Autodesk Inventor part; units mm, degrees
ref_plane "YZ Plane" through (0, 0, 0) normal (1, 0, 0) x (0, 1, 0)
ref_plane "XZ Plane" through (0, 0, 0) normal (0, 1, 0) x (-1, 0, 0)
ref_plane "XY Plane" through (0, 0, 0) normal (0, 0, 1) x (1, 0, 0)
sketch "Эскиз1" plane through (0, 0, 0) normal (0, 0, 1) x (1, 0, 0)
  arc A0 (0.9499, 0.3125) -> (0.1, 0.995) centre (0, 0) ccw
  line L0 (0.9499, 0.3125) -> (1.4499, 0.3125)
  line L1 (1.4499, 0.3125) -> (1.4499, -0.1875)
  line L2 (1.4499, -0.1875) -> (0.9823, -0.1875)
  arc A1 (0.1, -0.995) -> (0.9823, -0.1875) centre (0, 0) ccw
  line L3 (0.1, -0.995) -> (0.1, -4.5)
  line L4 (0.1, -4.5) -> (0.3, -4.7)
  line L5 (0.3, -4.7) -> (8.9, -4.7)
  line L6 (8.9, -4.7) -> (9.1, -4.5)
  line L7 (9.1, -4.5) -> (9.1, -0.995)
  arc A2 (8.2177, -0.1875) -> (9.1, -0.995) centre (9.2, 0) ccw
  line L8 (8.2177, -0.1875) -> (7.7501, -0.1875)
  line L9 (7.7501, -0.1875) -> (7.7501, 0.3125)
  line L10 (7.7501, 0.3125) -> (8.2501, 0.3125)
  arc A3 (9.1, 0.995) -> (8.2501, 0.3125) centre (9.2, 0) ccw
  line L11 (9.1, 0.995) -> (9.1, 1.6)
  line L12 (9.1, 1.6) -> (8.9, 1.8)
  line L13 (8.9, 1.8) -> (0.3, 1.8)
  line L14 (0.3, 1.8) -> (0.1, 1.6)
  line L15 (0.1, 1.6) -> (0.1, 0.995)
extrude "Выдавливание1" add sketch "Эскиз1" along normal blind 40
sketch "Эскиз2" plane through (0.3, 1.8, 0) normal (0, 1, 0) x (1, 0, 0)
  line L0 (4.3, -2.5) -> (4.3, -42.5) construction
  circle A0 centre (4.3, -10) radius 3
  line L1 (8.6, 0) -> (0, 0)
  dimension "d3" = 6
  dimension "d25" = 10
extrude "Выдавливание2" cut sketch "Эскиз2" against normal blind 3.5
sketch "Эскиз3" plane through (0.3, -4.7, 0) normal (0, -1, 0) x (1, 0, 0)
  line L0 (0, 0) -> (8.6, 0) construction
  line L1 (4.3, 0) -> (4.3, 8.2468) construction
  circle A0 centre (4.3, 10) radius 1.75
  point P0 (-0.3, 0)
  dimension "d26" = 3.5
  dimension "d27" = 10
extrude "Выдавливание3" cut sketch "Эскиз3" against normal blind 5
chamfer "Фаска1" distance 0.2 angle 45 2 edges at (2.85, -4.7, 10) (1.6, 1.8, 10)
pattern_linear "Прямоуг.массив1" count 2 spacing 20 along (0, 0, 1) of "Выдавливание3", "Выдавливание2", "Фаска1"
properties part number "рельса_мини"
Input: part model. Units: mm. Frame: model coordinates. A direction names the side the tool comes from. Round coordinates to 2 decimals unless told otherwise and drop trailing zeros. Order: outer loops, then holes, each group sorted by start corner. A loop starts at its lowest first (then second) coordinate and runs counter-clockwise, first axis right, second up. Notation, with made-up numbers: (9.25, 65.25) - (66.25, 65.25) arc R12 cw to (66.25, 87.25) - close; hole circle Ø2 at (-18.75, 29.5). An arc over 180 degrees is marked (long way). One line per question, with ' | ' between items. Start each with the question number.
1) Ray query, probe 1 along Z at (x, y) = (4.6, -3.3); probe 2 along Z at (x, y) = (4.6, -0.35); probe 3 along X at (y, z) = (0.1, 30). Return the intervals inside material, ascending.
2) Set-up query: faces 1 (the cylindrical face through (8.6, 0.8, 19.7)), 2 (the cylindrical face through (0.682, -0.732, 19.72)), 3 (the cylindrical face through (2.39, -0.03, 7.97)). Return all of +Z, -Z, +X, -X, +Y, -Y with unobstructed straight access to the full face (end or side cutting, diameter ignored); none if empty.
3) Contact query for flat-ended pins moving along their axis: P1, Ø2, axis at x = 1.5, z = 9.5, coming from the +Y side; P2, Ø3, axis at x = 5, z = 10.5, coming from the +Y side; P3, Ø0.6, axis at y = 0, z = 13, coming from the -X side; P4, Ø0.6, axis at y = 0, z = 23, coming from the +X side. Output: stop coordinate, or through.
4) Cut plane C-C, the plane y = -3. Return the cut outline in (x, z).
5) Pull-direction query (Z, two-part tool) for faces 4 (the flat face through (5, -1, 0)), 5 (the flat face through (5, -4.7, 20)), 6 (the cylindrical face through (5.41, -3.12, 28.45)); classes: +Z half, -Z half, draft (parallel to the pull), parting line (faces both ways), or undercut.
6) Cut plane A-A, the plane x = 4.6. Return the cut outline in (y, z), then the cut area to 3 significant figures.
Worked out:
1) probe 1: z = 0 to 8.25, 11.75 to 28.25, 31.75 to 40 | probe 2: z = 0 to 7, 13 to 27, 33 to 40 | probe 3: x = 1.45 to 1.6, 7.6 to 7.75
2) face 1: +Z, -Z, +X | face 2: +Z, -Z, -X | face 3: +Y
3) P1: stops at y = 1.8 | P2: stops at y = -1.7 | P3: stops at x = 0.95 | P4: stops at x = 8.25
4) outline: (0.1, 0) - (9.1, 0) - (9.1, 40) - (0.1, 40) - close; hole circle Ø3.5 at (4.6, 10); hole circle Ø3.5 at (4.6, 30)
5) face 4: -Z half | face 5: draft | face 6: undercut
6) outline: (-4.7, 0) - (1.8, 0) - (1.8, 6.8) - (1.6, 7) - (-1.7, 7) - (-1.7, 8.25) - (-4.5, 8.25) - (-4.7, 8.05) - close; (-4.7, 11.95) - (-4.5, 11.75) - (-1.7, 11.75) - (-1.7, 13) - (1.6, 13) - (1.8, 13.2) - (1.8, 26.8) - (1.6, 27) - (-1.7, 27) - (-1.7, 28.25) - (-4.5, 28.25) - (-4.7, 28.05) - close; (-4.7, 31.95) - (-4.5, 31.75) - (-1.7, 31.75) - (-1.7, 33) - (1.6, 33) - (1.8, 33.2) - (1.8, 40) - (-4.7, 40) - close | area: 197 mm^2
